Design review of the part shown in the three views and the two pictorial views. Dimensions are in mm from the part's minimum x, y and z. Coordinates: 2 decimals unless noted, no trailing zeros. Loops run counter-clockwise (first coordinate to the right, second up) from the corner with the lowest first, then second, coordinate; pieces in that order, holes last. Notation, with made-up numbers: (-32.75, 11) -> (-13.75, 11) arc R23 ccw to (-13.75, 20) -> close; hole circle Ø8 at (56, 28.25). An arc over 180 degrees is marked (long way). Answer in a Markdown table with one row per item.
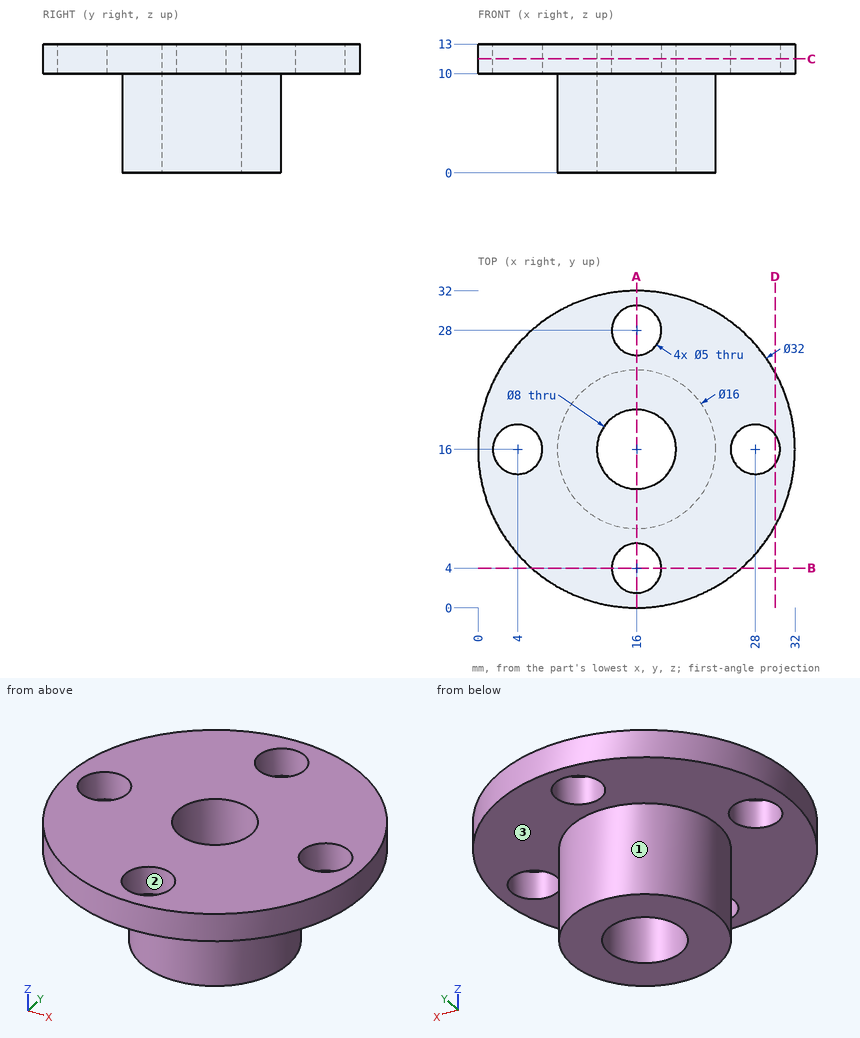
(1) Draft analysis for pull direction X (two halves, no side actions). For the marked faces 1, 2 and 3, state which applies: pulls with the +X half, pulls with the -X half, needs draft (parallel to the pull), parting line crosses it, or undercut.
Evaluation:
| item | result |
|---|---|
| face 1 | parting line crosses it |
| face 2 | undercut |
| face 3 | needs draft |
(2) For pin 1 (1.5 mm diameter, centred on x = 22.5, y = 6.5, fed in from -Z); pin 2 (3 mm diameter, centred on y = 14.5, z = 7.5, fed in from +X); pin 3 (1.5 mm diameter, centred on y = 20.5, z = 4.5, fed in from -X); pin 4 (6.5 mm diameter, centred on x = 16, y = 16, fed in from +Z), all flat-tipped, find the tip position at first contact; note any pin that passes through.
Evaluation:
| item | result |
|---|---|
| pin 1 | stops at z = 10 |
| pin 2 | stops at x = 24 |
| pin 3 | stops at x = 8.93 |
| pin 4 | passes through |
(3) Take a section at D-D on x = 30. Give the boundary of the cut face in (y, z).
Evaluation:
| item | result |
|---|---|
| outline | (8.25, 10) -> (14.5, 10) -> (14.5, 13) -> (8.25, 13) -> close; (17.5, 10) -> (23.75, 10) -> (23.75, 13) -> (17.5, 13) -> close |
(4) Take a section at B-B on y = 4. Give the boundary of the cut face in (x, z), and give its area (3 significant figures).
Evaluation:
| item | result |
|---|---|
| outline | (5.42, 10) -> (13.5, 10) -> (13.5, 13) -> (5.42, 13) -> close; (18.5, 10) -> (26.58, 10) -> (26.58, 13) -> (18.5, 13) -> close |
| area | 48.5 mm² |
(5) Take a section at C-C on z = 11.5. Give the boundary of the cut face in (x, y), and give its area (3 significant figures).
Evaluation:
| item | result |
|---|---|
| outline | circle Ø32 at (16, 16); hole circle Ø5 at (4, 16); hole circle Ø8 at (16, 16); hole circle Ø5 at (16, 4); hole circle Ø5 at (16, 28); hole circle Ø5 at (28, 16) |
| area | 675 mm² |
(6) Take a section at A-A on x = 16. Give the boundary of the cut face in (y, z).
Evaluation:
| item | result |
|---|---|
| outline | (0, 10) -> (1.5, 10) -> (1.5, 13) -> (0, 13) -> close; (6.5, 10) -> (8, 10) -> (8, 0) -> (12, 0) -> (12, 13) -> (6.5, 13) -> close; (20, 0) -> (24, 0) -> (24, 10) -> (25.5, 10) -> (25.5, 13) -> (20, 13) -> close; (30.5, 10) -> (32, 10) -> (32, 13) -> (30.5, 13) -> close |
(7) To check wall thickness, follow probe 1 along Y at (x, z) = (16, 11.6); probe 2 along Y at (x, z) = (16, 7.5); probe 3 along Z at (x, y) = (8.5, 28.5). State the ranges of each line that lie inside material, in increasing order.
Evaluation:
| item | result |
|---|---|
| probe 1 | y = 0 to 1.5, 6.5 to 12, 20 to 25.5, 30.5 to 32 |
| probe 2 | y = 8 to 12, 20 to 24 |
| probe 3 | z = 10 to 13 |
